Could you check a few things on this model? Use its own coordinates, in mm. A direction names the side the tool comes from. Coordinates: 2 decimals unless noted, no trailing zeros. Write each loop counter-clockwise with the first axis right and the second up, starting at its lowest first coordinate (ties: lowest second). Pieces come first, ordered by that corner, then holes.
```python
from build123d import *

# Parameters (mm, degrees)
F0_R     = 5
F1_DEPTH = 70
F2_R     = 7.5
F2_R_2   = 5
F3_DEPTH = 5
F4_R     = 2.5
F5_DEPTH = 25


with BuildPart() as f1:
    # F0 (on Top) → F1 (new body)
    with BuildSketch(Plane.XY):
        Circle(F0_R)
    extrude(amount=F1_DEPTH)

    # F2 (on face) → F3 (join)
    with BuildSketch(Plane(origin=(0, 0, 0), x_dir=(1, 0, 0), z_dir=(0, 0, -1))):
        Circle(F2_R)
        Circle(F2_R_2, mode=Mode.SUBTRACT)
        Circle(F2_R_2)
    extrude(amount=F3_DEPTH)

    # F4 (on face) → F5 (cut)
    with BuildSketch(Plane.XY.offset(70)):
        Circle(F4_R)
    extrude(amount=-F5_DEPTH, mode=Mode.SUBTRACT)


solid = f1.part
```
Item 1: I want a section at A-A, the plane y = 0. List the corners of the cut face in (x, z) for me.
Item 2: Which directions (+Z, -Z, +X, -X, +Y, -Y) give clear straight access to the entire face, cutting with the end or side of a thin tool? Please do faces 1 (the cylindrical face through (-7.493, -0.33, -2.465)), 2 (the flat face through (2, 5, 0)).
Item 3: I want a section at D-D, the plane x = 3.75. List the corners of the cut face in (y, z) for me, then the cut area to 3 significant figures.
Item 4: Will these pins go through, and if not, where does the flat tip stop? pin 1 Ø1 at (y, z) = (2, 53) entering from +X; pin 2 Ø2 at (y, z) = (-1, 9) entering from +X; pin 3 Ø3 at (y, z) = (2, 50) entering from -X.
Item 5: If I drill on line 1 along Y through (x, z) = (0, 54.25); line 2 along Z through (x, y) = (-1.75, 0.5); line 3 along Z through (x, y) = (0, 5.25), over which ranges is the centre line in solid material (lowest first)?
Item 6: If we mould it in two halves opening along Y, with no side actions, what happens to faces 3 (the flat face through (0, 0, 45)), 4 (the cylindrical face through (-0.54, -2.44, 57.68)), 5 (the cylindrical face through (-1.08, -4.88, 34.51)), 6 (the flat face through (2, -2, 70))? For each: released by +Y, released by -Y, zero draft, split by the parting line, or undercut.
Item 7: I want a section at C-C, the plane z = 34. List the corners of the cut face in (x, y) for me, then the cut area to 3 significant figures.
Taken from the geometry:
1. outline: (-7.5, -5) - (7.5, -5) - (7.5, 0) - (5, 0) - (5, 70) - (2.5, 70) - (2.5, 45) - (-2.5, 45) - (-2.5, 70) - (-5, 70) - (-5, 0) - (-7.5, 0) - close
2. face 1: +Z, -Z
2. face 2: +Z
3. outline: (-6.5, -5) - (6.5, -5) - (6.5, 0) - (3.31, 0) - (3.31, 70) - (-3.31, 70) - (-3.31, 0) - (-6.5, 0) - close
3. area: 528 mm2
4. pin 1: stops at x = 4.77
4. pin 2: stops at x = 5
4. pin 3: stops at x = -4.97
5. line 1: y = -5 to -2.5, 2.5 to 5
5. line 2: z = -5 to 45
5. line 3: z = -5 to 0
6. face 3: undercut
6. face 4: undercut
6. face 5: split by the parting line
6. face 6: zero draft
7. outline: circle Ø10 at (0, 0)
7. area: 78.5 mm2
